Work out the finished part from the listing and answer in its coordinate system (mm). Face numbers are marked on the shaded views. A direction names the side the tool comes from. Coordinates: 2 decimals unless noted, no trailing zeros. Write each loop counter-clockwise with the first axis right and the second up, starting at its lowest first coordinate (ties: lowest second). Pieces come first, ordered by that corner, then holes. Notation, with made-up numbers: M 51.5,31.5 L 103.5,31.5 A21 cw 103.5,35.5 Z; hole C 7,2 d7. An arc over 180 degrees is marked long. Use CSV: the item, a comma, the result in double quotes.
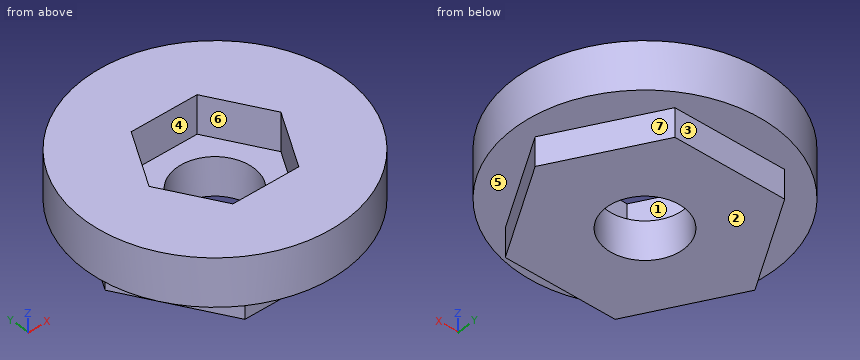
from build123d import *

# Parameters (mm, degrees)
BOSS_EXTRUDE1_DEPTH = 3
SKETCH3_R           = 13.5
BOSS_EXTRUDE2_DEPTH = 5
CUT_EXTRUDE1_DEPTH  = 4
SKETCH6_R           = 4
CUT_EXTRUDE2_DEPTH  = 9


with BuildPart() as part:
    # Sketch1 → Boss-Extrude1 (new body)
    with BuildSketch(Plane.XY):
        Polygon((11.547005384, 0), (5.773502692, 10), (-5.773502692, 10), (-11.547005384, 0), (-5.773502692, -10), (5.773502692, -10), align=None)
    extrude(amount=BOSS_EXTRUDE1_DEPTH)

    # Sketch3 → Boss-Extrude2 (add)
    with BuildSketch(Plane.XY.offset(3)):
        Circle(SKETCH3_R)
    extrude(amount=BOSS_EXTRUDE2_DEPTH)

    # Sketch4 → Cut-Extrude1 (cut)
    with BuildSketch(Plane.XY.offset(8)):
        Polygon((3.464101615, -6), (6.92820323, 0), (3.464101615, 6), (-3.464101615, 6), (-6.92820323, 0), (-3.464101615, -6), align=None)
    extrude(amount=-CUT_EXTRUDE1_DEPTH, mode=Mode.SUBTRACT)

    # Sketch6 → Cut-Extrude2 (cut, through all)
    with BuildSketch(Plane(origin=(0, 0, 0), x_dir=(-1, 0, 0), z_dir=(0, 0, -1))):
        Circle(SKETCH6_R)
    extrude(amount=-CUT_EXTRUDE2_DEPTH, mode=Mode.SUBTRACT)


solid = part.part
Item 1: The part is cut by section C-C (z = 6.75). Write down the section's boundary in (x, y), then the cut area to 3 significant figures.
Answer:
outline,"C 0,0 d27; hole M -6.93,0 L -3.46,-6 L 3.46,-6 L 6.93,0 L 3.46,6 L -3.46,6 Z"
area,"448 mm2"
Item 2: Given pin 1 (3.5 mm diameter, centred on x = 2, z = 2, fed in from -Y); pin 2 (7 mm diameter, centred on x = 0, y = 0, fed in from +Z); pin 3 (6 mm diameter, centred on x = 0, y = -1.5, fed in from +Z); pin 4 (1 mm diameter, centred on x = -3, z = 5.5, fed in from +Y), each flat-ended and moving along its own axis, determine where each tip first touches the part or whether it passes through.
Answer:
pin 1,"stops at y = -13.49"
pin 2,"passes through"
pin 3,"stops at z = 4"
pin 4,"stops at y = 13.27"
Item 3: The part is cut by section D-D (x = -9.75). Write down the section's boundary in (y, z).
Answer:
outline,"M -9.34,3 L -3.11,3 L -3.11,0 L 3.11,0 L 3.11,3 L 9.34,3 L 9.34,8 L -9.34,8 Z"
Item 4: Consider probe 1 along Y at (x, z) = (0, 2.65); probe 2 along Y at (x, z) = (0, 3.05); probe 3 along X at (y, z) = (-3, 5). Determine where each line is inside the solid, lowest interval first.
Answer:
probe 1,"y = -10 to -4, 4 to 10"
probe 2,"y = -13.5 to -4, 4 to 13.5"
probe 3,"x = -13.16 to -5.2, 5.2 to 13.16"
Item 5: The part is cut by section A-A (x = 0). Write down the section's boundary in (y, z), then the cut area to 3 significant figures.
Answer:
outline,"M -13.5,3 L -10,3 L -10,0 L -4,0 L -4,4 L -6,4 L -6,8 L -13.5,8 Z; M 4,0 L 10,0 L 10,3 L 13.5,3 L 13.5,8 L 6,8 L 6,4 L 4,4 Z"
area,"115 mm2"
Item 6: The part is cut by section B-B (y = -0.5). Write down the section's boundary in (x, z), then the cut area to 3 significant figures.
Answer:
outline,"M -13.49,3 L -11.26,3 L -11.26,0 L -3.97,0 L -3.97,4 L -6.64,4 L -6.64,8 L -13.49,8 Z; M 3.97,0 L 11.26,0 L 11.26,3 L 13.49,3 L 13.49,8 L 6.64,8 L 6.64,4 L 3.97,4 Z"
area,"118 mm2"
Item 7: A tool of negligible diameter and unlimited length cuts with its end or side. For the marked faces 5, 6 and 7, from which of +Z, -Z, +X, -X, +Y, -Y can it reach the whole face along a straight path? Write none if from no direction.
Answer:
face 5,"-Z"
face 6,"+Z"
face 7,"-Z, +X, +Y"
Item 8: For a pull along Y with two mould halves and no side action, classify the marked faces 1, 2, 3 and 4 as released by +Y, released by -Y, zero draft, split by the parting line, or undercut.
Answer:
face 1,"undercut"
face 2,"zero draft"
face 3,"released by +Y"
face 4,"undercut"
